The model under review builds one solid part; all positions refer to its coordinate system, in mm. A direction names the side the tool comes from. Give positions to 0.01 mm unless a question says otherwise; leave off trailing zeros. Order: outer loops, then holes, each group sorted by start corner. A loop starts at its lowest first (then second) coordinate and runs counter-clockwise, first axis right, second up.
```python
from build123d import *

# Parameters (mm, degrees)
F0_R     = 25.387749
F1_DEPTH = 25.4
F2_DEPTH = 12.7
F4_DEPTH = 25.4


with BuildPart() as f1:
    # F0 (on Top) → F1 (new body)
    with BuildSketch(Plane.XY):
        with BuildLine():
            Line((-31.190502, -14.275898), (0.254667, -14.275898))
            ThreePointArc((0.254667, -14.275898), (3.293439, -24.854389), (9.355083, -34.041069))
            ThreePointArc((9.355083, -34.041069), (72.758975, -9.630573), (9.355083, 14.779924))
            ThreePointArc((9.355083, 14.779924), (2.715424, 4.269314), (0, -7.862646))
            Line((0, -7.862646), (-31.190502, -7.862646))
            Line((-31.190502, -7.862646), (-31.190502, -14.275898))
        make_face()
        with Locations((36.358009, -9.630573)):
            Circle(F0_R, mode=Mode.SUBTRACT)
    extrude(amount=F1_DEPTH)

    # F0 (on Top) → F2 (join)
    with BuildSketch(Plane.XY):
        with BuildLine():
            ThreePointArc((9.355083, -34.041069), (3.293439, -24.854389), (0.254667, -14.275898))
            Line((0.254667, -14.275898), (-31.190502, -14.275898))
            Line((-31.190502, -14.275898), (-31.190502, -7.862646))
            Line((-31.190502, -7.862646), (0, -7.862646))
            ThreePointArc((0, -7.862646), (2.715424, 4.269314), (9.355083, 14.779924))
            Line((9.355083, 14.779924), (-45.523933, 14.779924))
            Line((-45.523933, 14.779924), (-45.523933, -32.019987))
            Line((-45.523933, -32.019987), (9.355083, -34.041069))
        make_face()
    extrude(amount=F2_DEPTH)

    # F3 (on face) → F4 (cut)
    with BuildSketch(Plane.XZ.offset(14.275898)):
        Polygon((-31.190502, 12.7), (0.254667, 25.4), (-31.190502, 25.4), align=None)
    extrude(amount=-F4_DEPTH, mode=Mode.SUBTRACT)


solid = f1.part
```
Item 1: Draft analysis for pull direction Y (two halves, no side actions). For faces 4 (the flat face through (-18, 14.78, 6)), 5 (the flat face through (-18, -4, 12.7)), 6 (the cylindrical face through (60.57, -2, 12.52)), 7 (the flat face through (-18.469, -33.016, 6.261)), state which applies: released by +Y, released by -Y, zero draft, split by the parting line, or undercut.
Values found:
face 4: released by +Y
face 5: zero draft
face 6: undercut
face 7: released by -Y
Item 2: Take a section at C-C (z = 19.75). Give the boundary of the cut face in (x, y).
Values found:
outline: (-13.73, -14.28) - (0.25, -14.28) arc R36.4 ccw to (9.36, -34.04) arc R36.4 ccw (long way) to (0, -7.86) - (-13.73, -7.86) - close; hole circle Ø50.78 at (36.36, -9.63)
Item 3: For line 1 (Z direction, x = -6, y = 11); line 2 (X direction, y = -8, z = 8); line 3 (X direction, y = 9.5, z = 21.5), list the stretches that pass through material, from the lowest coordinate up.
Values found:
line 1: z = 0 to 12.7
line 2: x = -45.52 to 11.02, 61.69 to 72.72
line 3: x = 5.39 to 19.67, 53.05 to 67.33
Item 4: Take a section at B-B (x = 33). Give the boundary of the cut face in (y, z).
Values found:
outline: (-45.88, 0) - (-34.8, 0) - (-34.8, 25.4) - (-45.88, 25.4) - close; (15.53, 0) - (26.62, 0) - (26.62, 25.4) - (15.53, 25.4) - close
Item 5: Take a section at A-A (y = -18.5). Give the boundary of the cut face in (x, z).
Values found:
outline: (-45.52, 0) - (12.57, 0) - (12.57, 25.4) - (1.05, 25.4) - (1.05, 12.7) - (-45.52, 12.7) - close; (60.15, 0) - (71.66, 0) - (71.66, 25.4) - (60.15, 25.4) - close
Item 6: Take a section at D-D (x = -36). Give the boundary of the cut face in (y, z), and give its area (3 significant figures).
Values found:
outline: (-32.37, 0) - (14.78, 0) - (14.78, 12.7) - (-32.37, 12.7) - close
area: 599 mm2
Item 7: For faces 1 (the flat face through (11.8, -17.2, 25.4)), 2 (the flat face through (-9, -14.276, 16)), 3 (the flat face through (-12, -7.863, 18)), list the 3-axis set-ups (+Z, -Z, +X, -X, +Y, -Y) from which the entire face can be reached by the end or side of a thin tool; tool diameter is ignored.
Values found:
face 1: +Z, +X, -X, +Y, -Y
face 2: +Z, -X, -Y
face 3: +Z, -X, +Y
Item 8: Clearance check with flat-ended pins moving along their axes: pin 1 Ø1.5 at (x, z) = (46, 8.5) entering from -Y; pin 2 Ø1.5 at (y, z) = (-32, 18) entering from +X; pin 3 Ø6.5 at (x, z) = (-12.5, 20) entering from +Y. State where each tip first meets the part, or that it passes through.
Values found:
pin 1: stops at y = -44.93
pin 2: stops at x = 65.64
pin 3: stops at y = -7.86
